from build123d import *

# Parameters (mm, degrees)
SKETCH1_R           = 1.25
SKETCH1_R_2         = 1.7
BOSS_EXTRUDE1_DEPTH = 3.5


with BuildPart() as part:
    # Sketch1 → Boss-Extrude1 (new body)
    with BuildSketch(Plane.XY):
        with BuildLine():
            Line((-30, -19), (30, -19))
            ThreePointArc((30, -19), (34, -15), (30, -11))
            Line((30, -11), (21.16, -11))
            ThreePointArc((21.16, -11), (13.381825407, -7.778174593), (10.16, 0))
            ThreePointArc((10.16, 0), (9.693763482, 1.54530035), (8.450656284, 2.574870238))
            ThreePointArc((8.450656284, 2.574870238), (7.225912675, 3.308465338), (6.253653028, 4.35387))
            ThreePointArc((6.253653028, 4.35387), (0, 7.619997387), (-6.253653028, 4.353870001))
            ThreePointArc((-6.253653028, 4.353870001), (-7.225911419, 3.308463788), (-8.450654495, 2.574865992))
            ThreePointArc((-8.450654495, 2.574865992), (-9.693759643, 1.545297801), (-10.159995392, 0))
            ThreePointArc((-10.159995392, 0), (-13.381820799, -7.778174593), (-21.159995392, -11))
            Line((-21.159995392, -11), (-30, -11))
            ThreePointArc((-30, -11), (-34, -15), (-30, -19))
        make_face()
        with Locations((-7.366, 0)):
            Circle(SKETCH1_R, mode=Mode.SUBTRACT)
        with Locations((7.366, 0)):
            Circle(SKETCH1_R, mode=Mode.SUBTRACT)
        with Locations((0, -15)):
            Circle(SKETCH1_R_2, mode=Mode.SUBTRACT)
        with BuildLine():
            Line((-30, -13.3), (-6, -13.3))
            ThreePointArc((-6, -13.3), (-4.3, -15), (-6, -16.7))
            Line((-6, -16.7), (-30, -16.7))
            ThreePointArc((-30, -16.7), (-31.7, -15), (-30, -13.3))
        make_face(mode=Mode.SUBTRACT)
        with BuildLine():
            Line((30, -16.7), (6, -16.7))
            ThreePointArc((6, -16.7), (4.3, -15), (6, -13.3))
            Line((6, -13.3), (30, -13.3))
            ThreePointArc((30, -13.3), (31.7, -15), (30, -16.7))
        make_face(mode=Mode.SUBTRACT)
    extrude(amount=BOSS_EXTRUDE1_DEPTH)


solid = part.part
Read the model definition and answer for the solid it produces. Units are mm, in the model's axes. A direction names the side the tool comes from. Give positions to 0.01 mm unless a question says otherwise; leave off trailing zeros. Loops run counter-clockwise (first coordinate to the right, second up) from the corner with the lowest first, then second, coordinate; pieces in that order, holes last. Notation, with made-up numbers: (74, 48) -> (114, 48) arc R8 cw to (114, 52) -> close; hole circle Ø10 at (-0.75, 2.25). An arc over 180 degrees is marked (long way). Use a Markdown table: item, result.
Q1. Section D-D, the plane x = -17.5 is taken. Determine the outline of the cut face in (y, z).
Solved:
| item | result |
|---|---|
| outline | (-19, 0) -> (-16.7, 0) -> (-16.7, 3.5) -> (-19, 3.5) -> close; (-13.3, 0) -> (-10.37, 0) -> (-10.37, 3.5) -> (-13.3, 3.5) -> close |
Q2. Section B-B, the plane y = -15 is taken. Determine the outline of the cut face in (x, z).
Solved:
| item | result |
|---|---|
| outline | (-34, 0) -> (-31.7, 0) -> (-31.7, 3.5) -> (-34, 3.5) -> close; (-4.3, 0) -> (-1.7, 0) -> (-1.7, 3.5) -> (-4.3, 3.5) -> close; (1.7, 0) -> (4.3, 0) -> (4.3, 3.5) -> (1.7, 3.5) -> close; (31.7, 0) -> (34, 0) -> (34, 3.5) -> (31.7, 3.5) -> close |
Q3. Section A-A, the plane x = 0 is taken. Determine the outline of the cut face in (y, z).
Solved:
| item | result |
|---|---|
| outline | (-19, 0) -> (-16.7, 0) -> (-16.7, 3.5) -> (-19, 3.5) -> close; (-13.3, 0) -> (7.62, 0) -> (7.62, 3.5) -> (-13.3, 3.5) -> close |
Q4. Determine the mould class of faces 4 (the face through (0, -8, 0)), 5 (the face through (-18, -16.7, 2)), 6 (the face through (-9.681, 1.564, 1.726)) for opening direction Y: pulls with the +Y half, pulls with the -Y half, needs draft (parallel to the pull), parting line crosses it, or undercut.
Solved:
| item | result |
|---|---|
| face 4 | needs draft |
| face 5 | undercut |
| face 6 | pulls with the +Y half |
Q5. A tool of negligible diameter and unlimited length cuts with its end or side. For faces 1 (the face through (-7.21, 3.32, 1.73)), 2 (the face through (26, -11, 2)), 3 (the face through (-18, -13.3, 2)), from which of +Z, -Z, +X, -X, +Y, -Y can it reach the whole face along a straight path? Write none if from no direction.
Solved:
| item | result |
|---|---|
| face 1 | +Z, -Z, -X, +Y |
| face 2 | +Z, -Z, +X, +Y |
| face 3 | +Z, -Z |
Q6. Each of these flat-tipped pins is pushed along its axis until it touches: pin 1 (8 mm diameter, centred on x = -6.5, y = -14.5, fed in from -Z); pin 2 (10 mm diameter, centred on x = -24.5, y = -3.5, fed in from +Z); pin 3 (1.5 mm diameter, centred on x = -2.5, z = 2.5, fed in from +Y); pin 4 (1 mm diameter, centred on x = -15, z = 1, fed in from +Y). Where does it stop, or does it pass through?
Solved:
| item | result |
|---|---|
| pin 1 | stops at z = 0 |
| pin 2 | passes through |
| pin 3 | stops at y = 7.42 |
| pin 4 | stops at y = -8.75 |
Q7. Find the intervals of material crossed by line 1 along Y through (x, z) = (-28, 1.8); line 2 along X through (y, z) = (-13.75, 0.35); line 3 along Y through (x, z) = (0, 2.55), in increasing order.
Solved:
| item | result |
|---|---|
| line 1 | y = -19 to -16.7, -13.3 to -11 |
| line 2 | x = -33.8 to -31.15, -4.85 to -1.15, 1.15 to 4.85, 31.15 to 33.8 |
| line 3 | y = -19 to -16.7, -13.3 to 7.62 |
Q8. Section C-C, the plane z = 1.05 is taken. Determine the outline of the cut face in (x, y).
Solved:
| item | result |
|---|---|
| outline | (-30, -19) -> (30, -19) arc R4 ccw to (30, -11) -> (21.16, -11) arc R11 cw to (10.16, 0) arc R2.79 ccw to (8.45, 2.57) arc R5.08 cw to (6.25, 4.35) arc R7.62 ccw to (-6.25, 4.35) arc R5.08 cw to (-8.45, 2.57) arc R2.79 ccw to (-10.16, 0) arc R11 cw to (-21.16, -11) -> (-30, -11) arc R4 ccw to start; hole (-30, -16.7) -> (-6, -16.7) arc R1.7 ccw to (-6, -13.3) -> (-30, -13.3) arc R1.7 ccw to start; hole circle Ø2.5 at (-7.37, 0); hole circle Ø3.4 at (0, -15); hole (6, -16.7) -> (30, -16.7) arc R1.7 ccw to (30, -13.3) -> (6, -13.3) arc R1.7 ccw to start; hole circle Ø2.5 at (7.37, 0) |
